Part model, mm, in its own coordinate system. Round coordinates to 2 decimals unless told otherwise and drop trailing zeros. Loops run counter-clockwise (first coordinate to the right, second up) from the corner with the lowest first, then second, coordinate; pieces in that order, holes last.
from build123d import *

# Parameters (mm, degrees)
BOSS_EXTRUDE1_DEPTH                   = 3.175
M3_CLEARANCE_HOLE1_D                  = 3.2
M3_CLEARANCE_HOLE1_CSINK_D            = 3.25
M3_CLEARANCE_HOLE1_CSINK_ANGLE        = 90
FILLET1_R                             = 10
FILLET2_R                             = 3
TAP_DRILL_FOR_M3X0_5_TAP2_D           = 2.5
TAP_DRILL_FOR_M3X0_5_TAP2_CSINK_D     = 2.55
TAP_DRILL_FOR_M3X0_5_TAP2_CSINK_ANGLE = 90
LPATTERN1_COUNT                       = 14
LPATTERN1_PITCH                       = 25


with BuildPart() as part:
    # Sketch1 → Boss-Extrude1 (new body)
    with BuildSketch(Plane(origin=(0, 0, 0), x_dir=(1, 0, 0), z_dir=(0, 1, 0))):
        Polygon((0, 0), (194, 0), (194, -2.7), (221, -2.7), (221, 29.7), (221, 35.5), (0, 35.5), (0, 29.7), align=None)
    extrude(amount=BOSS_EXTRUDE1_DEPTH)

    # M3 Clearance Hole1 (through all)
    with Locations(Plane(origin=(0, 3.175, 0), x_dir=(1, 0, 0), z_dir=(0, 1, 0))):
        with Locations((197.5, 21), (217.5, 6), (217.5, 21), (197.5, 6)):
            CounterSinkHole(M3_CLEARANCE_HOLE1_D / 2, M3_CLEARANCE_HOLE1_CSINK_D / 2, counter_sink_angle=M3_CLEARANCE_HOLE1_CSINK_ANGLE)

    # Fillet1
    # the kernel refuses this fillet: 10 mm, written as the material it adds along each edge
    with BuildSketch(Plane(origin=(194, 0, 0), x_dir=(-1, 0, 0), z_dir=(0, 1, 0))) as fillet1_piece_1:
        with BuildLine():
            CenterArc((6.83447145, 10), FILLET1_R, 226.886394054, 43.113605946)
            Line((0, 2.7), (-0.136689429, 2.554))
            ThreePointArc((-0.136689429, 2.554), (-0.2, 1.35), (-0.2, 0))
            Line((-0.2, 0), (0, -0.2))
            Line((0, -0.2), (6.83447145, -0.2))
            Line((6.83447145, -0.2), (6.83447145, 0))
        make_face()
    extrude(amount=3.175)

    # Fillet2
    fillet2_edges = [part.edges().sort_by_distance(p)[0] for p in [
        (221, 1.5875, -35.5),
        (221, 1.5875, 2.7),
        (194, 1.5875, 2.7),
    ]]
    fillet(fillet2_edges, radius=FILLET2_R)

    # Mirror1: part across plane


with BuildPart() as part_1:
    add(part.part)
    add(part.part.mirror(Plane(origin=(0, 3.175, -35.5), x_dir=(0, 0, 1), z_dir=(1, 0, 0))))

    # Tap Drill for M3x0.5 Tap2 (through all)
    with Locations(Plane(origin=(0, 0, 0), x_dir=(-1, 0, 0), z_dir=(0, -1, 0))):
        with Locations((166.5, 13.5)):
            tap_drill_for_m3x0_5_tap2 = CounterSinkHole(TAP_DRILL_FOR_M3X0_5_TAP2_D / 2, TAP_DRILL_FOR_M3X0_5_TAP2_CSINK_D / 2, counter_sink_angle=TAP_DRILL_FOR_M3X0_5_TAP2_CSINK_ANGLE)

    # LPattern1: Tap Drill for M3x0.5 Tap2 ×14
    with Locations(*[(i * LPATTERN1_PITCH, 0, 0) for i in range(1, LPATTERN1_COUNT)]):
        add(tap_drill_for_m3x0_5_tap2, mode=Mode.SUBTRACT)


solid = part_1.part
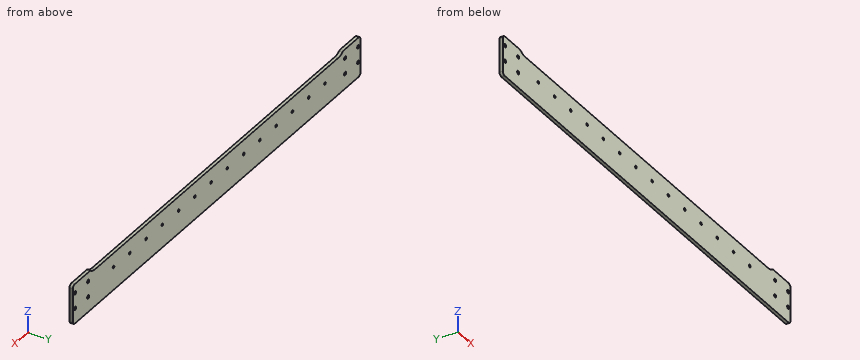
1) Slice it at B-B, the plane x = 93. Give the cut face in (y, z) (3 decimals).
Values:
outline: (0, -35.5) - (3.175, -35.5) - (3.175, 0) - (0, 0) - close
2) Drop a flat-ended pin along its axis: pin 1 Ø1 at (x, y) = (91, 2) entering from +Z. Give the stop position or say it passes through.
Values:
pin 1: stops at z = 0
3) Slice it at A-A, the plane y = 2.15. Give the number of separate pieces and of enclosed holes in the cut face, then the cut area to 3 significant figures.
Values:
separate pieces: 1
enclosed holes: 22
area: 15,700 mm2
4) Wall check: line 1 along X through (y, z) = (2.2, -6); line 2 along X through (y, z) = (2.5, -6.5); line 3 along Z through (x, y) = (-217.5, 2.35). Give the ranges that are in metal, low to high.
Values:
line 1: x = -221 to -219.1, -215.9 to -199.1, -195.9 to 195.9, 199.1 to 215.9, 219.1 to 221
line 2: x = -221 to -219.02, -215.98 to -199.02, -195.98 to 195.98, 199.02 to 215.98, 219.02 to 221
line 3: z = -35.5 to -22.6, -19.4 to -7.6, -4.4 to 2.7
